Check sheet for the modelled part. Datum: model origin and axes. Units: mm. A direction names the side the tool comes from. Coordinates: 2 decimals unless noted, no trailing zeros. Order: outer loops, then holes, each group sorted by start corner. A loop starts at its lowest first (then second) coordinate and runs counter-clockwise, first axis right, second up.
from build123d import *

# Parameters (mm, degrees)
F0_R     = 4
F0_R_2   = 2
F1_DEPTH = 1.5
F2_T     = -0.6
F3_DEPTH = 1.5
F4_T     = 0.6


# Not quite as in the source:
# - a shell that OpenCascade refuses in one call is made with other operations: the cavity is built on its own and cut out


with BuildPart() as f1:
    # F0 (on Top) → F1 (new body)
    with BuildSketch(Plane.XY):
        Circle(F0_R)
        Circle(F0_R_2, mode=Mode.SUBTRACT)
    extrude(amount=F1_DEPTH)

    # F2
    f2_openings = [f1.faces().sort_by_distance(p)[0] for p in [
        (-3.886863, 0, 1.5),
    ]]
    offset(amount=F2_T, openings=f2_openings)

    # F3 (add): a face of the model
    f3_faces = [f1.faces().sort_by_distance(p)[0] for p in [
        (-3.886862915, 0, 0),
    ]]
    extrude(f3_faces, amount=F3_DEPTH)

    # F4: shell of thickness 0.6, made by hand


with BuildPart() as f4_core1:
    # F4_t2: copy of F1
    add(f1.part)

    # the walls: a layer under each face that stays
    f4_faces = [f4_core1.faces().sort_by_distance(p)[0] for p in [
        (-4, 0, 0.75),
        (-4, 0, -0.75),
        (-2.6666666667, -2.6666666667, 1.5),
        (-3.4, 0, 1.05),
        (-2, 0, -0.75),
        (-2.2666666667, -2.2666666667, 0.6),
        (-2, 0, 0.75),
        (-2.6, 0, 1.05),
        (-1.7333333333, -1.7333333333, 1.5),
    ]]
    thicken(f4_faces, amount=-F4_T, mode=Mode.SUBTRACT)

    # F4_s3 → F4_t4 (revolve, cut)
    with BuildSketch(Plane.XZ):
        Polygon((3.394, 0.606), (4, 0.6), (4, 0), (3.4, 0), align=None)
    revolve(axis=Axis((0, 0, 0.6), (0, 0, -1)), mode=Mode.SUBTRACT)

    # F4_s5 → F4_t6 (revolve, cut)
    with BuildSketch(Plane.XZ):
        Polygon((2.606, 0.606), (2.6, 0), (2, 0), (2, 0.6), align=None)
    revolve(axis=Axis((0, 0, 0.6), (0, 0, -1)), mode=Mode.SUBTRACT)


with BuildPart() as f1_1:
    add(f1.part)

    # what is left inside the walls is the cavity
    f4_cavity = [f4_core1.part.solids().sort_by_distance(p)[0] for p in [
        (-3.394, 0, -1),
    ]]
    add(f4_cavity, mode=Mode.SUBTRACT)


solid = f1_1.part
(1) Cross-section at C-C (z = 0.75). Enter the section's corners in (x, y).
Filled in:
outline: circle Ø8 at (0, 0); circle Ø5.2 at (0, 0); hole circle Ø6.8 at (0, 0); hole circle Ø4 at (0, 0)
(2) Tool access check on faces 1 (the flat face through (-2, -3, 1.5)), 2 (the cylindrical face through (-0.74, -3.32, -0.74)), 3 (the cylindrical face through (-0.74, -3.32, 1.04)). Record the directions out of +Z, -Z, +X, -X, +Y, -Y that give a thin tool (end or side, any length) a straight path to the whole face; none if there is none.
Filled in:
face 1: +Z, +X, -X, +Y, -Y
face 2: -Z
face 3: +Z
(3) Thickness scan on probe 1 along Y at (x, z) = (0, 0.8); probe 2 along X at (y, z) = (0.75, 0.85). Record the ranges inside material, lowest first.
Filled in:
probe 1: y = -4 to -3.4, -2.6 to -2, 2 to 2.6, 3.4 to 4
probe 2: x = -3.93 to -3.32, -2.49 to -1.85, 1.85 to 2.49, 3.32 to 3.93
(4) Go/stop test with a flat-tipped pin: P1, Ø3, axis at x = -2, y = -2, coming from the +Z side. Record where the tip stops, or that it passes through.
Filled in:
P1: stops at z = 1.5
(5) Cross-section at A-A (x = 0). Enter the section's corners in (y, z), and give its area (3 significant figures).
Filled in:
outline: (-4, -1.5) - (-3.4, -1.5) - (-3.4, 0) - (-2.6, 0) - (-2.6, -1.5) - (-2, -1.5) - (-2, 1.5) - (-2.6, 1.5) - (-2.6, 0.6) - (-3.4, 0.6) - (-3.4, 1.5) - (-4, 1.5) - close; (2, -1.5) - (2.6, -1.5) - (2.6, 0) - (3.4, 0) - (3.4, -1.5) - (4, -1.5) - (4, 1.5) - (3.4, 1.5) - (3.4, 0.6) - (2.6, 0.6) - (2.6, 1.5) - (2, 1.5) - close
area: 8.16 mm2
(6) Cross-section at D-D (y = 3). Enter the section's corners in (x, z).
Filled in:
outline: (-2.65, -1.5) - (-1.6, -1.5) - (-1.6, 0) - (1.6, 0) - (1.6, -1.5) - (2.65, -1.5) - (2.65, 1.5) - (1.6, 1.5) - (1.6, 0.6) - (-1.6, 0.6) - (-1.6, 1.5) - (-2.65, 1.5) - close
(7) Release check for a two-part mould opening along Y. For faces 4 (the flat face through (-1, -3, 0.6)), 5 (the flat face through (1, -2, -1.5)), 6 (the cylindrical face through (-0.338, 2.578, 1.044)), 7 (the cylindrical face through (-0.867, -3.905, 0.021)) record: +Y half, -Y half, draft (parallel to the pull), parting line (faces both ways), or undercut.
Filled in:
face 4: undercut
face 5: draft
face 6: undercut
face 7: parting line
